Read the model definition and answer for the solid it produces. Units are mm, in the model's axes. Face numbers are marked on the shaded views. A direction names the side the tool comes from. Coordinates: 2 decimals unless noted, no trailing zeros. Order: outer loops, then holes, each group sorted by start corner. A loop starts at its lowest first (then second) coordinate and runs counter-clockwise, first axis right, second up. Notation, with made-up numbers: (31.25, 86) - (53.25, 86) arc R14 cw to (53.25, 90) - close; hole circle Ø2 at (35, 4). An arc over 180 degrees is marked (long way). Write item = value, one per line.
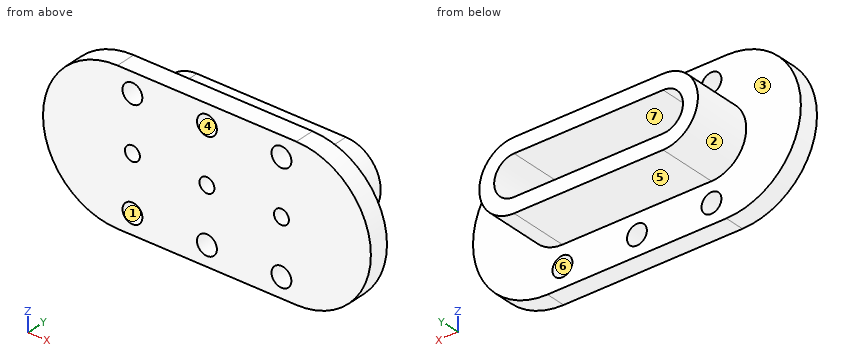
from build123d import *

# Parameters (mm, degrees)
BOSS_EXTRUDE1_DEPTH = 10
BOSS_EXTRUDE2_DEPTH = 60
HOLE1_D             = 20
HOLE2_D             = 15


with BuildPart() as part:
    # Sketch1 → Boss-Extrude1 (new, symmetric)
    with BuildSketch(Plane(origin=(0, 0, 0), x_dir=(1, 0, 0), z_dir=(0, 1, 0))):
        with BuildLine():
            Line((-90, 75), (90, 75))
            ThreePointArc((90, 75), (165, 0), (90, -75))
            Line((90, -75), (-90, -75))
            ThreePointArc((-90, -75), (-165, 0), (-90, 75))
        make_face()
    extrude(amount=BOSS_EXTRUDE1_DEPTH, both=True)

    # Sketch2 → Boss-Extrude2 (add)
    with BuildSketch(Plane(origin=(0, 10, 0), x_dir=(1, 0, 0), z_dir=(0, 1, 0))):
        with BuildLine():
            Line((-75, 35), (75, 35))
            ThreePointArc((75, 35), (110, 0), (75, -35))
            Line((75, -35), (-75, -35))
            ThreePointArc((-75, -35), (-110, 0), (-75, 35))
        make_face()
        with BuildLine():
            Line((-75, 20), (75, 20))
            ThreePointArc((75, 20), (95, 0), (75, -20))
            Line((75, -20), (-75, -20))
            ThreePointArc((-75, -20), (-95, 0), (-75, 20))
        make_face(mode=Mode.SUBTRACT)
    extrude(amount=BOSS_EXTRUDE2_DEPTH)

    # Hole1 (through all)
    with Locations(Plane(origin=(0, 10, 0), x_dir=(1, 0, 0), z_dir=(0, 1, 0))):
        with Locations((75, -55), (0, -55), (-75, -55)):
            hole1 = Hole(HOLE1_D / 2)

    # Mirror1: Hole1 across plane
    add(hole1.mirror(Plane.XY), mode=Mode.SUBTRACT)

    # Hole2 (through all)
    with Locations(Plane(origin=(0, 10, 0), x_dir=(1, 0, 0), z_dir=(0, 1, 0))):
        with Locations((0, 0), (75, 0), (-75, 0)):
            Hole(HOLE2_D / 2)


solid = part.part
1) The part is cut by section B-B (z = 55). Determine the outline of the cut face in (x, y).
Returned:
outline = (-140.99, -10) - (-85, -10) - (-85, 10) - (-140.99, 10) - close; (-65, -10) - (-10, -10) - (-10, 10) - (-65, 10) - close; (10, -10) - (65, -10) - (65, 10) - (10, 10) - close; (85, -10) - (140.99, -10) - (140.99, 10) - (85, 10) - close
2) Flat-ended cylindrical pins translate along their axes: pin 1 Ø13.5 at (x, z) = (0, 0) entering from +Y; pin 2 Ø12 at (x, z) = (-118.5, -49) entering from +Y; pin 3 Ø3 at (x, y) = (100, 40.5) entering from -Z; pin 4 Ø4 at (x, y) = (17, 12.5) entering from -Z. Find the tip coordinate at first contact, or state that the pin passes through.
Returned:
pin_1 = through
pin_2 = 10
pin_3 = -25.94
pin_4 = -35
3) The part is cut by section A-A (y = -3.5). Count the separate pieces of the cut face and the enclosed holes in it, and give its area (3 significant figures).
Returned:
separate_pieces = 1
enclosed_holes = 9
area = 42,300 mm^2
4) Straight lines are drawn through the part: line 1 along Z through (x, y) = (75, 1.5); line 2 along Z through (x, y) = (-42, 41); line 3 along X through (y, z) = (4, -49). For each, find the intervals that lie inside material, in ascending order. Write a range as from..to.
Returned:
line_1 = -75..-65, -45..-7.5, 7.5..45, 65..75
line_2 = -35..-20, 20..35
line_3 = -146.78..-83, -67..-8, 8..67, 83..146.78
5) For the marked faces 5, 6 and 7, determine the directions among +Z, -Z, +X, -X, +Y, -Y from which every point of the face is accessible in a straight line to the end or side of a thin tool.
Returned:
face_5 = -Z, +X, -X, +Y
face_6 = +Y, -Y
face_7 = +Y
6) The part is cut by section D-D (x = 18.5). Determine the outline of the cut face in (y, z), and give its area (3 significant figures).
Returned:
outline = (-10, -75) - (10, -75) - (10, -35) - (70, -35) - (70, -20) - (10, -20) - (10, 20) - (70, 20) - (70, 35) - (10, 35) - (10, 75) - (-10, 75) - close
area = 4,800 mm^2
7) The part is cut by section C-C (y = 31.5). Determine the outline of the cut face in (x, z), and give its area (3 significant figures).
Returned:
outline = (-75, -35) - (75, -35) arc R35 ccw to (75, 35) - (-75, 35) arc R35 ccw to start; hole (-75, -20) - (75, -20) arc R20 ccw to (75, 20) - (-75, 20) arc R20 ccw to start
area = 7,090 mm^2
8) Determine the mould class of the marked faces 1, 2, 3 and 4 for opening direction Z: pulls with the +Z half, pulls with the -Z half, needs draft (parallel to the pull), parting line crosses it, or undercut.
Returned:
face_1 = undercut
face_2 = parting line crosses it
face_3 = needs draft
face_4 = undercut
